Answer from the drawing. Dimensions are ordinates in mm from the lowest x, y and z of the part. A direction names the side the tool comes from. Give positions to 0.01 mm unless a question says otherwise; leave off trailing zeros. Loops run counter-clockwise (first coordinate to the right, second up) from the corner with the lowest first, then second, coordinate; pieces in that order, holes last. Notation, with made-up numbers: (-15, 80.5) - (36, 80.5) arc R22 ccw to (36, 106.5) - close; hole circle Ø4 at (-12, 10). An arc over 180 degrees is marked (long way). One line per item, written item: value.
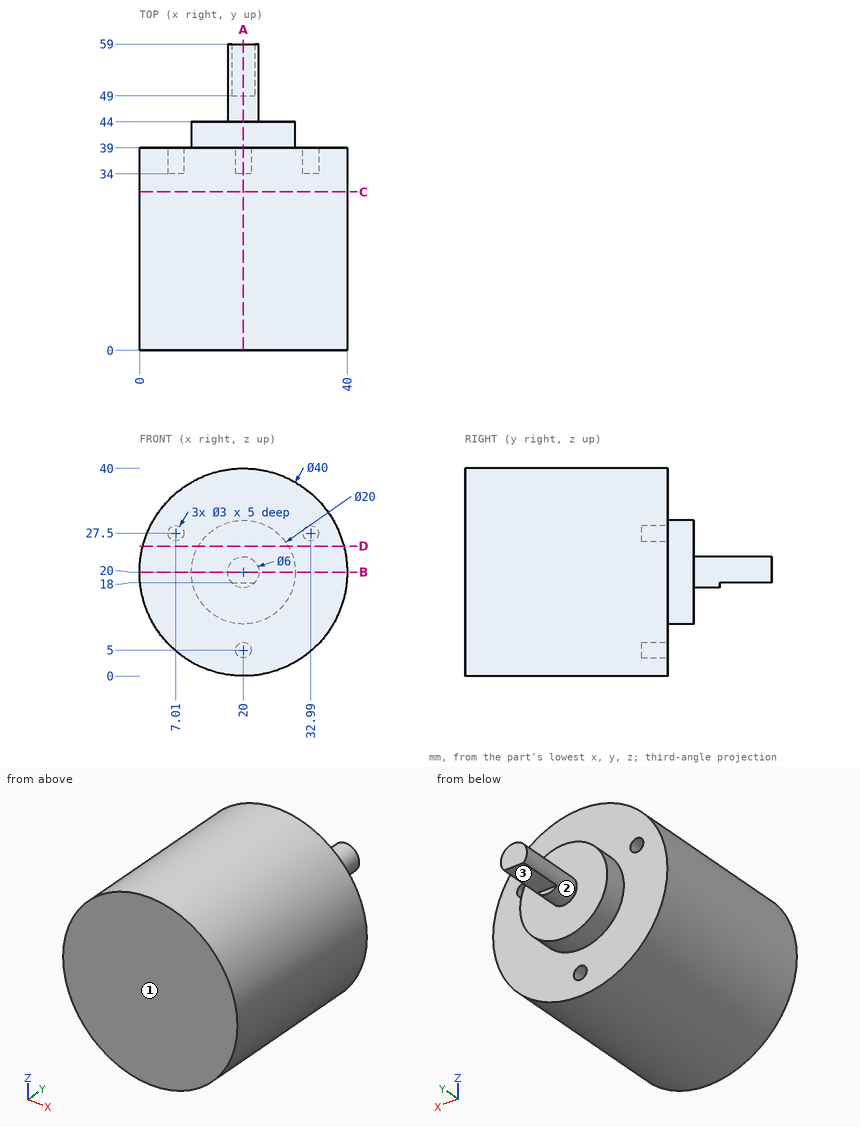
1. Section D-D (z = 25) is taken. Write down the section's boundary in (x, y) (1 decimal).
Output:
outline: (0.6, 0) - (39.4, 0) - (39.4, 39) - (28.7, 39) - (28.7, 44) - (11.3, 44) - (11.3, 39) - (0.6, 39) - close
2. Flat-ended cylindrical pins translate along their axes: pin 1 Ø0.9 at (x, z) = (19.5, 5) entering from +Y; pin 2 Ø10 at (x, y) = (5, 15.5) entering from +Z; pin 3 Ø1 at (x, z) = (28, 25.5) entering from +Y; pin 4 Ø8 at (y, z) = (44.5, 6) entering from -X. Find the tip coordinate at first contact, or state that the pin passes through.
Output:
pin 1: stops at y = 34
pin 2: stops at z = 37.32
pin 3: stops at y = 44
pin 4: passes through
3. Section C-C (y = 30.5) is taken. Write down the section's boundary in (x, z), and give its area (3 significant figures).
Output:
outline: circle Ø40 at (20, 20)
area: 1,260 mm²
4. Find the intervals of material crossed by line 1 along Y through (x, z) = (13, 6); line 2 along Y through (x, z) = (21, 11); line 3 along X through (y, z) = (37, 27) (1 decimal), in increasing order.
Output:
line 1: y = 0 to 39
line 2: y = 0 to 44
line 3: x = 1.3 to 5.6, 8.4 to 31.6, 34.4 to 38.7
5. Section B-B (z = 20) is taken. Write down the section's boundary in (x, y), and give its area (3 significant figures).
Output:
outline: (0, 0) - (40, 0) - (40, 39) - (30, 39) - (30, 44) - (23, 44) - (23, 59) - (17, 59) - (17, 44) - (10, 44) - (10, 39) - (0, 39) - close
area: 1,750 mm²
6. For the marked faces 1, 2 and 3, determine the directions among +Z, -Z, +X, -X, +Y, -Y from which every point of the face is accessible in a straight line to the end or side of a thin tool.
Output:
face 1: +Z, -Z, +X, -X, -Y
face 2: +Y
face 3: -Z, +X, -X, +Y
7. Section A-A (x = 20) is taken. Write down the section's boundary in (y, z), and give its area (4 significant figures).
Output:
outline: (0, 0) - (39, 0) - (39, 3.5) - (34, 3.5) - (34, 6.5) - (39, 6.5) - (39, 10) - (44, 10) - (44, 17) - (49, 17) - (49, 18) - (59, 18) - (59, 23) - (44, 23) - (44, 30) - (39, 30) - (39, 40) - (0, 40) - close
area: 1,725 mm²
